from build123d import *

# Parameters (mm, degrees)
SKETCH1_R                = 16.002
BOSS_EXTRUDE1_DEPTH      = 6.35
SKETCH2_W                = 50.8
SKETCH2_H                = 8.255
BOSS_EXTRUDE2_DEPTH      = 15.875
FILLET1_R                = 5.08
CHAMFER1_SIZE            = 3.175
SKETCH3_R                = 2.921
CUT_EXTRUDE1_DEPTH       = 72.867301501
FILLET1_OF_MIRROR2_R     = 5.08
CHAMFER1_OF_MIRROR2_SIZE = 3.175


with BuildPart() as part:
    # Sketch1 → Boss-Extrude1 (new body)
    with BuildSketch(Plane(origin=(0, 0, 0), x_dir=(0, 0, -1), z_dir=(1, 0, 0))):
        with BuildLine():
            Line((0, 0), (50.8, 0))
            Line((50.8, 0), (50.8, 34.925))
            ThreePointArc((50.8, 34.925), (45.220384182, 48.395384182), (31.75, 53.975))
            Line((31.75, 53.975), (19.05, 53.975))
            ThreePointArc((19.05, 53.975), (5.579615818, 48.395384182), (0, 34.925))
            Line((0, 34.925), (0, 0))
        make_face()
        with Locations((25.4, 30.48)):
            Circle(SKETCH1_R, mode=Mode.SUBTRACT)
    boss_extrude1 = extrude(amount=BOSS_EXTRUDE1_DEPTH)

    # Sketch2 → Boss-Extrude2 (add)
    with BuildSketch(Plane(origin=(6.35, 0, 0), x_dir=(0, 0, -1), z_dir=(1, 0, 0))):
        with Locations((25.4, 4.1275)):
            Rectangle(SKETCH2_W, SKETCH2_H)
    boss_extrude2 = extrude(amount=BOSS_EXTRUDE2_DEPTH)

    # Fillet1
    fillet1_edges = [part.edges().sort_by_distance(p)[0] for p in [
        (6.35, 8.255, -25.4),
    ]]
    fillet(fillet1_edges, radius=FILLET1_R)

    # Chamfer1
    chamfer1_edges = [part.edges().sort_by_distance(p)[0] for p in [
        (6.35, 48.395384182, -45.220384182),
        (6.35, 53.975, -25.4),
        (16.8275, 8.255, 0),
        (6.35, 48.395384182, -5.579615818),
        (16.8275, 8.255, -50.8),
        (22.225, 4.1275, 0),
        (22.225, 4.1275, -50.8),
        (22.225, 8.255, -25.4),
        (6.35, 24.13, -50.8),
        (7.837897552, 9.742897552, 0),
        (7.837897552, 9.742897552, -50.8),
        (6.35, 24.13, 0),
    ]]
    chamfer(chamfer1_edges, length=CHAMFER1_SIZE)

    # Sketch3 → Cut-Extrude1 (cut, through all)
    with BuildSketch(Plane(origin=(0, 8.255, 0), x_dir=(1, 0, 0), z_dir=(0, 1, 0))):
        with Locations(Location((15.24, 9.525, 0), (0, 0, 270))):
            Circle(SKETCH3_R)
        with Locations(Location((15.24, 41.275, 0), (0, 0, 90))):
            Circle(SKETCH3_R)
    cut_extrude1 = extrude(amount=-CUT_EXTRUDE1_DEPTH, mode=Mode.SUBTRACT)

    # Mirror2: Boss-Extrude1, Boss-Extrude2, Cut-Extrude1 across plane
    add(boss_extrude1.mirror(Plane(origin=(0, 34.925, -19.05), x_dir=(0, 0, 1), z_dir=(1, 0, 0))))
    add(boss_extrude2.mirror(Plane(origin=(0, 34.925, -19.05), x_dir=(0, 0, 1), z_dir=(1, 0, 0))))
    add(cut_extrude1.mirror(Plane(origin=(0, 34.925, -19.05), x_dir=(0, 0, 1), z_dir=(1, 0, 0))), mode=Mode.SUBTRACT)

    # Fillet1 of Mirror2
    fillet1_of_mirror2_edges = [part.edges().sort_by_distance(p)[0] for p in [
        (-6.35, 8.255, -25.4),
    ]]
    fillet(fillet1_of_mirror2_edges, radius=FILLET1_OF_MIRROR2_R)

    # Chamfer1 of Mirror2
    chamfer1_of_mirror2_edges = [part.edges().sort_by_distance(p)[0] for p in [
        (-6.35, 48.395384182, -45.220384182),
        (-6.35, 53.975, -25.4),
        (-16.8275, 8.255, 0),
        (-6.35, 48.395384182, -5.579615818),
        (-16.8275, 8.255, -50.8),
        (-22.225, 4.1275, 0),
        (-22.225, 4.1275, -50.8),
        (-22.225, 8.255, -25.4),
        (-6.35, 24.13, -50.8),
        (-7.837897552, 9.742897552, 0),
        (-7.837897552, 9.742897552, -50.8),
        (-6.35, 24.13, 0),
    ]]
    chamfer(chamfer1_of_mirror2_edges, length=CHAMFER1_OF_MIRROR2_SIZE)


solid = part.part
The model under review builds one solid part; all positions refer to its coordinate system, in mm. A direction names the side the tool comes from. Give positions to 0.01 mm unless a question says otherwise; leave off trailing zeros. Order: outer loops, then holes, each group sorted by start corner. A loop starts at its lowest first (then second) coordinate and runs counter-clockwise, first axis right, second up. Notation, with made-up numbers: M -2.5,63 L 8.5,63 A13 ccw 8.5,72 Z; hole C 44,-2 d1. An arc over 180 degrees is marked long. Use one line per item in the form item = value. Start each with the question number.
Item 1: Insertion check: pin 1 Ø6.5 at (x, z) = (-15.24, -41.275) entering from +Y (3 decimals); pin 2 Ø5 at (y, z) = (11.5, -5.5) entering from -X; pin 3 Ø8 at (y, z) = (26, -37) entering from -X; pin 4 Ø10 at (y, z) = (7.5, -41.5) entering from -X (3 decimals). Each pin has a flat end and moves straight along its axis. Give the tip position at first contact, or say it passes through.
Item 2: We need section B-B on x = -15.24. Give the boundary of the cut face in (y, z) (3 decimals), plus the area to 3 significant figures.
Item 3: To check wall thickness, follow line 1 along Z through (x, y) = (-15.24, 3.25); line 2 along Z through (x, y) = (-15.24, 6.5); line 3 along Z through (x, y) = (-3, 30). State the ranges of each line that lie inside material, in increasing order. Write a range as from..to.
Item 4: We need section C-C on z = -25.4. Give the boundary of the cut face in (x, y) (3 decimals).
Item 5: We need section A-A on y = 30.48. Give the boundary of the cut face in (x, z) (3 decimals), plus the area to 3 significant figures.
Item 6: For faces 1 (the flat face through (15.19, 6.65, -1.57)), 2 (the flat face through (-4.74, 24.281, -1.565)), 3 (the flat face through (15, 8.255, -25)), list the 3-axis set-ups (+Z, -Z, +X, -X, +Y, -Y) from which the entire face can be reached by the end or side of a thin tool; tool diameter is ignored.
Item 7: We need section D-D on x = 1. Give the boundary of the cut face in (y, z) (3 decimals).
Completed:
q1.pin_1 = 8.255
q1.pin_2 = -8.78
q1.pin_3 = -6.35
q1.pin_4 = -22.225
q2.outline = M 0,-50.8 L 5.08,-50.8 L 8.255,-47.625 L 8.255,-44.196 L 0,-44.196 Z; M 0,-38.354 L 8.255,-38.354 L 8.255,-12.446 L 0,-12.446 Z; M 0,-6.604 L 8.255,-6.604 L 8.255,-3.175 L 5.08,0 L 0,0 Z
q2.area = 313 mm²
q3.line_1 = -50.8..-44.2, -38.35..-12.45, -6.6..0
q3.line_2 = -49.38..-44.2, -38.35..-12.45, -6.6..-1.42
q3.line_3 = -50.8..-41.39, -9.41..0
q4.outline = M -22.225,0 L 22.225,0 L 22.225,5.08 L 19.05,8.255 L 11.43,8.255 A5.08 cw 6.35,13.335 L 6.35,14.478 L -6.35,14.478 L -6.35,13.335 A5.08 cw -11.43,8.255 L -19.05,8.255 L -22.225,5.08 Z; M -6.35,46.482 L 6.35,46.482 L 6.35,50.8 L 3.175,53.975 L -3.175,53.975 L -6.35,50.8 Z
q5.outline = M -6.35,-47.625 L -3.175,-50.8 L 3.175,-50.8 L 6.35,-47.625 L 6.35,-41.402 L -6.35,-41.402 Z; M -6.35,-9.398 L 6.35,-9.398 L 6.35,-3.175 L 3.175,0 L -3.175,0 L -6.35,-3.175 Z
q5.area = 219 mm²
q6.face_1 = +Z, +X, +Y
q6.face_2 = +Z, -X, +Y
q6.face_3 = +Z, -Z, +X, +Y
q7.outline = M 0,-50.8 L 34.925,-50.8 A19.05 ccw 53.975,-31.75 L 53.975,-19.05 A19.05 ccw 34.925,0 L 0,0 Z; hole C 30.48,-25.4 d32.004
